For this review, use the dimensioned drawing (mm, ordinates from the lowest corner) and the shaded views. Coordinates: 2 decimals unless noted, no trailing zeros. Loops run counter-clockwise (first coordinate to the right, second up) from the corner with the lowest first, then second, coordinate; pieces in that order, holes last. Notation, with made-up numbers: M 52,5.5 L 81,5.5 A19 ccw 81,36.5 Z; hole C 55,58 d4. An arc over 180 degrees is marked long. One line per item, written item: value.
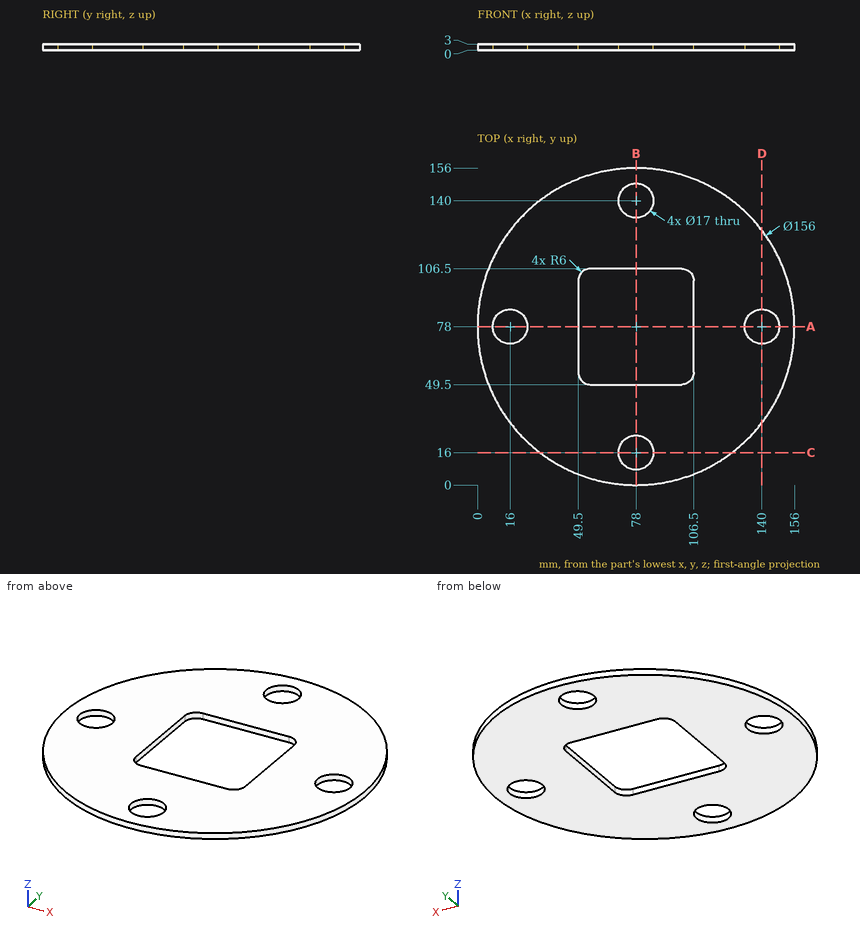
(1) We need section A-A on y = 78. State the section outline as (x, z) points.
Reply:
outline: M 0,0 L 7.5,0 L 7.5,3 L 0,3 Z; M 24.5,0 L 49.5,0 L 49.5,3 L 24.5,3 Z; M 106.5,0 L 131.5,0 L 131.5,3 L 106.5,3 Z; M 148.5,0 L 156,0 L 156,3 L 148.5,3 Z
(2) We need section C-C on y = 16. State the section outline as (x, z) points, then the cut area to 3 significant figures.
Reply:
outline: M 30.67,0 L 69.5,0 L 69.5,3 L 30.67,3 Z; M 86.5,0 L 125.33,0 L 125.33,3 L 86.5,3 Z
area: 233 mm2
(3) To check wall thickness, follow line 1 along Y through (x, z) = (78.5, 2.4); line 2 along X through (y, z) = (85, 0.85); line 3 along Y through (x, z) = (79.5, 1.4). State the ranges of each line that lie inside material, in increasing order. Write a range as [from, to].
Reply:
line 1: y = [0, 7.51], [24.49, 49.5], [106.5, 131.51], [148.49, 156]
line 2: x = [0.31, 11.18], [20.82, 49.5], [106.5, 135.18], [144.82, 155.69]
line 3: y = [0.01, 7.63], [24.37, 49.5], [106.5, 131.63], [148.37, 155.99]
(4) Insertion check: pin 1 (2 mm diameter, centred on x = 37.5, y = 48, fed in from -Z); pin 2 (1 mm diameter, centred on y = 83.5, z = 0.5, fed in from -X); pin 3 (0.9 mm diameter, centred on y = 70, z = 2, fed in from -X); pin 4 (1 mm diameter, centred on y = 102.5, z = 1.5, fed in from +X). Each pin has a flat end and moves straight along its axis. Give the tip position at first contact, or say it passes through.
Reply:
pin 1: stops at z = 0
pin 2: stops at x = 0.16
pin 3: stops at x = 0.37
pin 4: stops at x = 152.22
